The listing builds one solid part. Answer for the finished solid, in the listing's coordinates (mm). A direction names the side the tool comes from. Give positions to 0.01 mm unless a question says otherwise; leave off trailing zeros. Loops run counter-clockwise (first coordinate to the right, second up) from the corner with the lowest first, then second, coordinate; pieces in that order, holes last. Notation, with made-up numbers: (-6.5, 88) - (-1.5, 88) arc R22 ccw to (-1.5, 104) - close; hole circle Ø6 at (52, 39.5). An arc over 180 degrees is marked (long way). Write each question's results on one line, items separated by ' | '.
from build123d import *

# Parameters (mm, degrees)
F0_R     = 18.5
F0_R_2   = 1.5
F0_R_3   = 3
F1_DEPTH = 55
F2_R     = 5
F3_DEPTH = 4
F4_R     = 3
F5_DEPTH = 12


with BuildPart() as f1:
    # F0 (on Front) → F1 (new body)
    with BuildSketch(Plane.XZ):
        Circle(F0_R)
        with Locations((-15.5, 0)):
            Circle(F0_R_2, mode=Mode.SUBTRACT)
        with Locations((0, 7)):
            Circle(F0_R_3, mode=Mode.SUBTRACT)
        with Locations((15.5, 0)):
            Circle(F0_R_2, mode=Mode.SUBTRACT)
    extrude(amount=F1_DEPTH)

    # F2 (on face) → F3 (join)
    with BuildSketch(Plane.XZ.offset(55)):
        with Locations((0, 7)):
            Circle(F2_R)
    extrude(amount=F3_DEPTH)

    # F4 (on face) → F5 (join)
    with BuildSketch(Plane.XZ.offset(59)):
        with Locations((0, 7)):
            Circle(F4_R)
    extrude(amount=F5_DEPTH)


solid = f1.part
Item 1: A cutting plane is placed at A-A, the plane x = 15.5. Determine the outline of the cut face in (y, z), plus the area to 3 significant figures.
Values found:
outline: (-55, -10.1) - (0, -10.1) - (0, -1.5) - (-55, -1.5) - close; (-55, 1.5) - (0, 1.5) - (0, 10.1) - (-55, 10.1) - close | area: 946 mm²
Item 2: Find the intervals of material crossed by line 1 along X through (y, z) = (-12.5, 0.5); line 2 along Y through (x, z) = (-12, 0.5); line 3 along Z through (x, y) = (15, -39), in increasing order. Write a range as [from, to].
Values found:
line 1: x = [-18.49, -16.91], [-14.09, 14.09], [16.91, 18.49] | line 2: y = [-55, 0] | line 3: z = [-10.83, -1.41], [1.41, 10.83]
Item 3: Flat-ended cylindrical pins translate along their axes: P1, Ø8, axis at x = 13, y = -30.5, coming from the -Z side; P2, Ø1, axis at y = -36, z = -1.5, coming from the -X side; P3, Ø3, axis at x = 0, z = 6.5, coming from the +Y side. Find the tip coordinate at first contact, or state that the pin passes through.
Values found:
P1: stops at z = -16.16 | P2: stops at x = -18.47 | P3: stops at y = -55
Item 4: For faces 1 (the face through (-3, -27, 7)), 2 (the face through (0, 0, 0)), 3 (the face through (-3, -65, 7)), determine the directions among +Z, -Z, +X, -X, +Y, -Y from which every point of the face is accessible in a straight line to the end or side of a thin tool.
Values found:
face 1: +Y | face 2: +Z, -Z, +X, -X, +Y | face 3: -Y
Item 5: A cutting plane is placed at D-D, the plane y = -17. Determine the outline of the cut face in (x, z).
Values found:
outline: circle Ø37 at (0, 0); hole circle Ø3 at (-15.5, 0); hole circle Ø6 at (0, 7); hole circle Ø3 at (15.5, 0)
Item 6: A cutting plane is placed at C-C, the plane x = 0. Determine the outline of the cut face in (y, z).
Values found:
outline: (-71, 4) - (-59, 4) - (-59, 2) - (-55, 2) - (-55, -18.5) - (0, -18.5) - (0, 4) - (-55, 4) - (-55, 10) - (0, 10) - (0, 18.5) - (-55, 18.5) - (-55, 12) - (-59, 12) - (-59, 10) - (-71, 10) - close
Item 7: A cutting plane is placed at B-B, the plane z = 7. Determine the outline of the cut face in (x, y), plus the area to 3 significant figures.
Values found:
outline: (-17.12, -55) - (-5, -55) - (-5, -59) - (-3, -59) - (-3, -71) - (3, -71) - (3, -59) - (5, -59) - (5, -55) - (17.12, -55) - (17.12, 0) - (3, 0) - (3, -55) - (-3, -55) - (-3, 0) - (-17.12, 0) - close | area: 1,670 mm²
Item 8: For a pull along X with two mould halves and no side action, classify faces 4 (the face through (-4.01, -27.12, -18.06)), 5 (the face through (0, -71, 7)), 6 (the face through (0, -55, 7)) as released by +X, released by -X, zero draft, split by the parting line, or undercut.
Values found:
face 4: split by the parting line | face 5: zero draft | face 6: undercut
